Input: dimensioned drawing with shaded views. Units: mm. Origin: part minimum x, y, z. Coordinates: 2 decimals unless noted, no trailing zeros. Order: outer loops, then holes, each group sorted by start corner. A loop starts at its lowest first (then second) coordinate and runs counter-clockwise, first axis right, second up. Notation, with made-up numbers: (46, -39) -> (89, -39) arc R18 cw to (89, -30) -> close; hole circle Ø3 at (54.5, -25.5). An arc over 180 degrees is marked (long way). Answer as CSV lines item,"result".
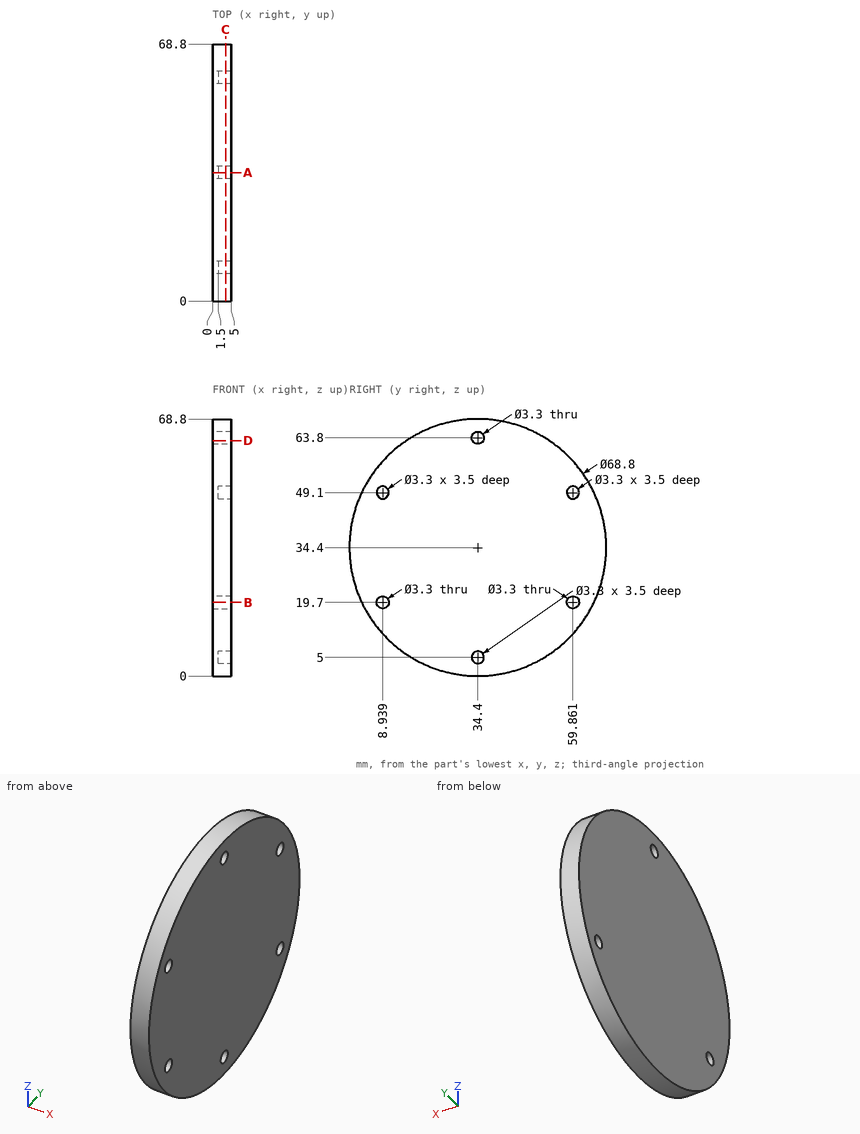
1. Ray query, line 1 along Y through (x, z) = (2.2, 19.7); line 2 along Z through (x, y) = (2.3, 9); line 3 along Z through (x, y) = (3.3, 59.5). Return the intervals inside material, ascending.
Findings:
line 1,"y = 3.3 to 7.29, 10.59 to 58.21, 61.51 to 65.5"
line 2,"z = 11.2 to 18.05, 21.35 to 47.45, 50.75 to 57.6"
line 3,"z = 10.88 to 18.09, 21.31 to 47.49, 50.71 to 57.92"
2. Contact query for flat-ended pins moving along their axis: pin 1 (2 mm diameter, centred on y = 8.94, z = 49.1, fed in from +X); pin 2 (3 mm diameter, centred on x = 4, y = 49, fed in from -Z); pin 3 (1 mm diameter, centred on x = 4, z = 10.5, fed in from -Y) (1 decimal). Output: stop coordinate, or through.
Findings:
pin 1,"stops at x = 1.5"
pin 2,"stops at z = 2.59"
pin 3,"stops at y = 9.2"
3. Cut plane B-B (z = 19.7). Return the cut outline in (x, y).
Findings:
outline,"(0, 3.3) -> (5, 3.3) -> (5, 7.29) -> (0, 7.29) -> close; (0, 10.59) -> (5, 10.59) -> (5, 58.21) -> (0, 58.21) -> close; (0, 61.51) -> (5, 61.51) -> (5, 65.5) -> (0, 65.5) -> close"
4. Cut plane C-C (x = 3.5). Return the cut outline in (y, z), plus the area to 3 significant figures.
Findings:
outline,"circle Ø68.8 at (34.4, 34.4); hole circle Ø3.3 at (8.94, 19.7); hole circle Ø3.3 at (8.94, 49.1); hole circle Ø3.3 at (34.4, 5); hole circle Ø3.3 at (34.4, 63.8); hole circle Ø3.3 at (59.86, 19.7); hole circle Ø3.3 at (59.86, 49.1)"
area,"3,670 mm2"
5. Cut plane A-A (y = 34.4). Return the cut outline in (x, z).
Findings:
outline,"(0, 0) -> (5, 0) -> (5, 3.35) -> (1.5, 3.35) -> (1.5, 6.65) -> (5, 6.65) -> (5, 62.15) -> (0, 62.15) -> close; (0, 65.45) -> (5, 65.45) -> (5, 68.8) -> (0, 68.8) -> close"
6. Cut plane D-D (z = 63). Return the cut outline in (x, y), plus the area to 3 significant figures.
Findings:
outline,"(0, 15.28) -> (5, 15.28) -> (5, 32.96) -> (0, 32.96) -> close; (0, 35.84) -> (5, 35.84) -> (5, 53.52) -> (0, 53.52) -> close"
area,"177 mm2"
